```python
from build123d import *

# Parameters (mm, degrees)
SKETCH1_W               = 210
SKETCH1_H               = 210
MAINEXTRUDE_DEPTH       = 4
SKETCH1_6_R             = 1.5
SCREWHOLES_DEPTH        = 4
ROUNDEDCORNERS_R        = 10
SKETCH3_R               = 7
SKETCH3_R_2             = 1.5
SKETCH3_W               = 136
SKETCH3_H               = 10
TRENCH_DEPTH            = 10
SKETCH4_W               = 140
SKETCH4_H               = 14
SKETCH4_W_2             = 136
SKETCH4_H_2             = 10
TRENCH_WALLS_DEPTH      = 4
SKETCH5_W               = 140
SKETCH5_H               = 14
TRENCH_BOTTOM_DEPTH     = 2
SKETCH7_W               = 10
SKETCH7_H               = 6
WIRE_OPENING_DEPTH      = 36
WIRE_OPENING_DEPTH_BACK = 176
SKETCH9_R               = 2
SKETCH9_R_2             = 0.98
PCB_HOLES_DEPTH         = 4
PCB_ROUNDS_R            = 2


with BuildPart() as part:
    # Sketch1 → MainExtrude (new body)
    with BuildSketch(Plane(origin=(0, 0, 0), x_dir=(1, 0, 0), z_dir=(0, 1, 0))):
        Rectangle(SKETCH1_W, SKETCH1_H)
    extrude(amount=MAINEXTRUDE_DEPTH)

    # Sketch1_6 → ScrewHoles (cut)
    with BuildSketch(Plane(origin=(0, 0, 0), x_dir=(1, 0, 0), z_dir=(0, 1, 0))):
        with Locations((-99.833273811, 99.833273811)):
            Circle(SKETCH1_6_R)
        with Locations((-99.833273811, -99.833273811)):
            Circle(SKETCH1_6_R)
        with Locations((99.833273811, -99.833273811)):
            Circle(SKETCH1_6_R)
        with Locations((99.833273811, 99.833273811)):
            Circle(SKETCH1_6_R)
    extrude(amount=SCREWHOLES_DEPTH, mode=Mode.SUBTRACT)

    # RoundedCorners
    roundedcorners_edges = [part.edges().sort_by_distance(p)[0] for p in [
        (-105, 2, -105),
        (-105, 2, 105),
        (105, 2, 105),
        (105, 2, -105),
    ]]
    fillet(roundedcorners_edges, radius=ROUNDEDCORNERS_R)

    # Sketch3 → Trench (cut)
    with BuildSketch(Plane(origin=(0, 0, 0), x_dir=(1, 0, 0), z_dir=(0, 1, 0))):
        with Locations((0, -80)):
            Circle(SKETCH3_R)
        with Locations((-9, -68)):
            Circle(SKETCH3_R_2)
        with Locations((-9, -94.3)):
            Circle(SKETCH3_R_2)
        with Locations((10.8, -94.3)):
            Circle(SKETCH3_R_2)
        with Locations((10.8, -68)):
            Circle(SKETCH3_R_2)
        with Locations((0, 79.5)):
            Rectangle(SKETCH3_W, SKETCH3_H)
        with Locations((0, 62.5)):
            Rectangle(SKETCH3_W, SKETCH3_H)
        with Locations((0, 45.5)):
            Rectangle(SKETCH3_W, SKETCH3_H)
        with Locations((0, 28.5)):
            Rectangle(SKETCH3_W, SKETCH3_H)
        with Locations((0, 11.5)):
            Rectangle(SKETCH3_W, SKETCH3_H)
        with Locations((0, -5.5)):
            Rectangle(SKETCH3_W, SKETCH3_H)
        with Locations((0, -22.5)):
            Rectangle(SKETCH3_W, SKETCH3_H)
        with Locations((0, -39.5)):
            Rectangle(SKETCH3_W, SKETCH3_H)
    extrude(amount=TRENCH_DEPTH, mode=Mode.SUBTRACT)

    # Sketch4 → Trench Walls (add)
    with BuildSketch(Plane(origin=(0, 0, 0), x_dir=(1, 0, 0), z_dir=(0, 1, 0))):
        with Locations((0, 79.5)):
            Rectangle(SKETCH4_W, SKETCH4_H)
        with Locations((0, 79.5)):
            Rectangle(SKETCH4_W_2, SKETCH4_H_2, mode=Mode.SUBTRACT)
        with Locations((0, 62.5)):
            Rectangle(SKETCH4_W, SKETCH4_H)
        with Locations((0, 62.5)):
            Rectangle(SKETCH4_W_2, SKETCH4_H_2, mode=Mode.SUBTRACT)
        with Locations((0, 45.5)):
            Rectangle(SKETCH4_W, SKETCH4_H)
        with Locations((0, 45.5)):
            Rectangle(SKETCH4_W_2, SKETCH4_H_2, mode=Mode.SUBTRACT)
        with Locations((0, 28.5)):
            Rectangle(SKETCH4_W, SKETCH4_H)
        with Locations((0, 28.5)):
            Rectangle(SKETCH4_W_2, SKETCH4_H_2, mode=Mode.SUBTRACT)
        with Locations((0, 11.5)):
            Rectangle(SKETCH4_W, SKETCH4_H)
        with Locations((0, 11.5)):
            Rectangle(SKETCH4_W_2, SKETCH4_H_2, mode=Mode.SUBTRACT)
        with Locations((0, -5.5)):
            Rectangle(SKETCH4_W, SKETCH4_H)
        with Locations((0, -5.5)):
            Rectangle(SKETCH4_W_2, SKETCH4_H_2, mode=Mode.SUBTRACT)
        with Locations((0, -22.5)):
            Rectangle(SKETCH4_W, SKETCH4_H)
        with Locations((0, -22.5)):
            Rectangle(SKETCH4_W_2, SKETCH4_H_2, mode=Mode.SUBTRACT)
        with Locations((0, -39.5)):
            Rectangle(SKETCH4_W, SKETCH4_H)
        with Locations((0, -39.5)):
            Rectangle(SKETCH4_W_2, SKETCH4_H_2, mode=Mode.SUBTRACT)
    extrude(amount=-TRENCH_WALLS_DEPTH)

    # Sketch5 → Trench Bottom (add)
    with BuildSketch(Plane.XZ.offset(4)):
        with Locations((0, -79.5)):
            Rectangle(SKETCH5_W, SKETCH5_H)
        with Locations((0, -62.5)):
            Rectangle(SKETCH5_W, SKETCH5_H)
        with Locations((0, -45.5)):
            Rectangle(SKETCH5_W, SKETCH5_H)
        with Locations((0, -28.5)):
            Rectangle(SKETCH5_W, SKETCH5_H)
        with Locations((0, -11.5)):
            Rectangle(SKETCH5_W, SKETCH5_H)
        with Locations((0, 5.5)):
            Rectangle(SKETCH5_W, SKETCH5_H)
        with Locations((0, 22.5)):
            Rectangle(SKETCH5_W, SKETCH5_H)
        with Locations((0, 39.5)):
            Rectangle(SKETCH5_W, SKETCH5_H)
    extrude(amount=TRENCH_BOTTOM_DEPTH)

    # Sketch7 → Wire Opening (cut, two sides)
    with BuildSketch(Plane(origin=(70, 0, 0), x_dir=(0, 0, -1), z_dir=(1, 0, 0))) as wire_opening_sk:
        with Locations((-39.5, -3)):
            Rectangle(SKETCH7_W, SKETCH7_H)
        with Locations((-22.5, -3)):
            Rectangle(SKETCH7_W, SKETCH7_H)
        with Locations((-5.5, -3)):
            Rectangle(SKETCH7_W, SKETCH7_H)
        with Locations((11.5, -3)):
            Rectangle(SKETCH7_W, SKETCH7_H)
        with Locations((28.5, -3)):
            Rectangle(SKETCH7_W, SKETCH7_H)
        with Locations((45.5, -3)):
            Rectangle(SKETCH7_W, SKETCH7_H)
        with Locations((62.5, -3)):
            Rectangle(SKETCH7_W, SKETCH7_H)
        with Locations((79.5, -3)):
            Rectangle(SKETCH7_W, SKETCH7_H)
    extrude(amount=WIRE_OPENING_DEPTH, mode=Mode.SUBTRACT)
    extrude(wire_opening_sk.sketch, amount=-WIRE_OPENING_DEPTH_BACK, mode=Mode.SUBTRACT)

    # Sketch9 → PCB Holes (add)
    with BuildSketch(Plane.XZ):
        with Locations((-94, 92)):
            Circle(SKETCH9_R)
        with Locations((-94, 92)):
            Circle(SKETCH9_R_2, mode=Mode.SUBTRACT)
        with Locations((-19.73, 92)):
            Circle(SKETCH9_R)
        with Locations((-19.73, 92)):
            Circle(SKETCH9_R_2, mode=Mode.SUBTRACT)
        with Locations((-94, 56.16)):
            Circle(SKETCH9_R)
        with Locations((-94, 56.16)):
            Circle(SKETCH9_R_2, mode=Mode.SUBTRACT)
        with Locations((-19.73, 56.16)):
            Circle(SKETCH9_R)
        with Locations((-19.73, 56.16)):
            Circle(SKETCH9_R_2, mode=Mode.SUBTRACT)
    extrude(amount=PCB_HOLES_DEPTH)

    # PCB Rounds
    pcb_rounds_edges = [part.edges().sort_by_distance(p)[0] for p in [
        (-96, 0, 92),
        (-21.73, 0, 56.16),
        (-96, 0, 56.16),
        (-21.73, 0, 92),
    ]]
    fillet(pcb_rounds_edges, radius=PCB_ROUNDS_R)


solid = part.part
```
Source: CAD feature listing. Evaluate the final solid. Frame: model axes, mm. A direction names the side the tool comes from. Round coordinates to 2 decimals unless told otherwise and drop trailing zeros. Loops run counter-clockwise (first coordinate to the right, second up) from the corner with the lowest first, then second, coordinate; pieces in that order, holes last. Notation, with made-up numbers: (-18, 33) - (41, 33) arc R30 cw to (41, 61) - close; hole circle Ø5 at (9.5, -3). An arc over 180 degrees is marked (long way). Use CSV: the item, a comma, the result in double quotes.
Q1. Reachability of faces 1 (the cylindrical face through (101.99, 2.03, 102.15)), 2 (the flat face through (-1, -3, -86.5)), 3 (the flat face through (-1, -3, -35.5)) from +Z, -Z, +X, -X, +Y, -Y: full face, straight path, thin tool, end or side. Return the list, or none.
Reported:
face 1,"+Z, +X, +Y, -Y"
face 2,"-Z, +X, -X, -Y"
face 3,"+X, -X, -Y"
Q2. Mould query, pull axis X, two halves, no side actions, for faces 4 (the cylindrical face through (-102.15, 2.03, -101.99)), 5 (the flat face through (-1, -3, -38.5)), 6 (the flat face through (1, -1, -16.5)). Classes: pulls with the +X half, pulls with the -X half, needs draft (parallel to the pull), parting line crosses it, or undercut.
Reported:
face 4,"pulls with the -X half"
face 5,"needs draft"
face 6,"undercut"
Q3. Section query C-C, the plane z = 7. Output: boundary loops of the cut face in (x, y), then the cut area to 3 significant figures.
Reported:
outline,"(-105, 0) - (-68, 0) - (-68, 4) - (-105, 4) - close; (68, 0) - (105, 0) - (105, 4) - (68, 4) - close"
area,"296 mm^2"
Q4. Section query A-A, the plane z = 80. Output: boundary loops of the cut face in (x, y), then the cut area to 3 significant figures.
Reported:
outline,"(-105, 0) - (-7, 0) - (-7, 4) - (-105, 4) - close; (7, 0) - (105, 0) - (105, 4) - (7, 4) - close"
area,"784 mm^2"
Q5. Section query B-B, the plane x = 56.5. Give the number of separate pieces and of enclosed holes in the cut face, then the cut area to 3 significant figures.
Reported:
separate pieces,"9"
enclosed holes,"0"
area,"712 mm^2"
Q6. Ray query, line 1 along X through (y, z) = (2.65, 68); line 2 along Z through (x, y) = (-94, -2.15); line 3 along X through (y, z) = (0.5, -45.5). Return the intervals inside material, ascending.
Reported:
line 1,"-105 to -10.5, -7.5 to 9.3, 12.3 to 105"
line 2,"54.16 to 55.18, 57.14 to 58.16, 90 to 91.02, 92.98 to 94"
line 3,"-105 to -68, 68 to 105"
Q7. Pin query (flat end, axial travel): pin 1 Ø2.5 at (x, z) = (99.83, -99.83) entering from -Y; pin 2 Ø1.6 at (y, z) = (-4, -86) entering from -X; pin 3 Ø2 at (y, z) = (-2.5, -5) entering from +X; pin 4 Ø1.5 at (x, y) = (-28, -3) entering from -Z. Return the tip coordinate at first contact, or that it passes through.
Reported:
pin 1,"through"
pin 2,"x = -70"
pin 3,"x = 70"
pin 4,"z = -86.5"
